from build123d import *

# Parameters (mm, degrees)
BOSS_EXTRUDE1_DEPTH = 40
SKETCH2_R           = 2
CUT_EXTRUDE1_DEPTH  = 7.1
SKETCH9_R           = 1
CUT_EXTRUDE2_DEPTH  = 4.1


with BuildPart() as part:
    # Sketch1 → Boss-Extrude1 (new body)
    with BuildSketch(Plane.XY):
        Polygon((-2.460653528, 0), (2.460653528, 0), (5.25, 2.789346472), (5.25, 4.3), (3.065, 4.3), (4.865, 6.1), (-4.865, 6.1), (-3.065, 4.3), (-5.25, 4.3), (-5.25, 2.789346472), align=None)
    extrude(amount=BOSS_EXTRUDE1_DEPTH)

    # Sketch2 → Cut-Extrude1 (cut, through all)
    with BuildSketch(Plane(origin=(0, 6.1, 0), x_dir=(1, 0, 0), z_dir=(0, 1, 0))):
        with Locations((0, -30)):
            Circle(SKETCH2_R)
        with Locations((0, -10)):
            Circle(SKETCH2_R)
    extrude(amount=-CUT_EXTRUDE1_DEPTH, mode=Mode.SUBTRACT)

    # Sketch9 → Cut-Extrude2 (cut)
    with BuildSketch(Plane(origin=(0, 6.1, 0), x_dir=(1, 0, 0), z_dir=(0, 1, 0))):
        with Locations((-3.065, -35)):
            Circle(SKETCH9_R)
        with Locations((-3.065, -25)):
            Circle(SKETCH9_R)
    extrude(amount=-CUT_EXTRUDE2_DEPTH, mode=Mode.SUBTRACT)


solid = part.part
Could you check a few things on this model? Use its own coordinates, in mm. A direction names the side the tool comes from. Give positions to 0.01 mm unless a question says otherwise; leave off trailing zeros. Write each loop counter-clockwise with the first axis right and the second up, starting at its lowest first coordinate (ties: lowest second). Pieces come first, ordered by that corner, then holes. Notation, with made-up numbers: (-23.5, -29.5) -> (6.5, -29.5) arc R16 ccw to (6.5, -11.5) -> close; hole circle Ø5 at (-8.5, 37.25). An arc over 180 degrees is marked (long way). Answer as CSV lines item,"result". Start each with the question number.
(1) If we section it at B-B, the plane x = 0: Write out the boundary of the cut face in (y, z).
(2) If we section it at D-D, the plane y = 1.5: Write out the boundary of the cut face in (x, z), and give its area (3 significant figures).
(3) If we mould it in two halves opening along Y, with no side actions, what happens to faces 1 (the face through (0, 6.1, 20)), 2 (the face through (-3.978, 5.213, 19.72)), 3 (the face through (4, 4.3, 20)), 4 (the face through (0, 3, 32))? For each: +Y half, -Y half, draft (parallel to the pull), parting line (faces both ways), or undercut.
(4) I'm going to push a flat-ended pin straight in: pin 1 Ø2.5 at (x, z) = (0, 10) entering from -Y. Where does the tip first touch, or does it pass through?
(5) If we section it at C-C, the plane z = 25: Write out the boundary of the cut face in (x, y) (3 decimals).
(6) Which directions (+Z, -Z, +X, -X, +Y, -Y) give clear straight access to the entire face, cutting with the end or side of a thin tool? Please do faces 5 (the face through (-3, 2, 35)), 6 (the face through (0, 3, 0)), 7 (the face through (3.952, 5.187, 19.72)).
(7) If we section it at A-A, the plane z = 30: Write out the boundary of the cut face in (x, y) (3 decimals), and give its area (3 significant figures).
(8) Please list where these lines run through material, in increasing order: line 1 (Z direction, x = 0, y = 4.5); line 2 (Z direction, x = -1.5, y = 1.5); line 3 (X direction, y = 3.55, z = 25) (3 decimals).
Answer list:
1,outline,"(0, 0) -> (6.1, 0) -> (6.1, 8) -> (0, 8) -> close; (0, 12) -> (6.1, 12) -> (6.1, 28) -> (0, 28) -> close; (0, 32) -> (6.1, 32) -> (6.1, 40) -> (0, 40) -> close"
2,outline,"(-3.96, 0) -> (3.96, 0) -> (3.96, 40) -> (-3.96, 40) -> close; hole circle Ø4 at (0, 10); hole circle Ø4 at (0, 30)"
2,area,"292 mm^2"
3,face 1,"+Y half"
3,face 2,"undercut"
3,face 3,"undercut"
3,face 4,"draft"
4,pin 1,"through"
5,outline,"(-5.25, 2.789) -> (-2.461, 0) -> (2.461, 0) -> (5.25, 2.789) -> (5.25, 4.3) -> (3.065, 4.3) -> (4.865, 6.1) -> (-2.065, 6.1) -> (-2.065, 2) -> (-4.065, 2) -> (-4.065, 4.3) -> (-5.25, 4.3) -> close; (-4.865, 6.1) -> (-4.065, 5.3) -> (-4.065, 6.1) -> close"
6,face 5,"+Y"
6,face 6,"-Z, +X, -X, +Y, -Y"
6,face 7,"+Z, -Z, +X"
7,outline,"(-5.25, 2.789) -> (-2.461, 0) -> (-2, 0) -> (-2, 6.1) -> (-4.865, 6.1) -> (-3.065, 4.3) -> (-5.25, 4.3) -> close; (2, 0) -> (2.461, 0) -> (5.25, 2.789) -> (5.25, 4.3) -> (3.065, 4.3) -> (4.865, 6.1) -> (2, 6.1) -> close"
7,area,"27.2 mm^2"
8,line 1,"0 to 8, 12 to 28, 32 to 40"
8,line 2,"0 to 8.68, 11.32 to 28.68, 31.32 to 40"
8,line 3,"-5.25 to -4.065, -2.065 to 5.25"
